Input: dimensioned drawing with shaded views. Units: mm. Origin: part minimum x, y, z. Round coordinates to 2 decimals unless told otherwise and drop trailing zeros. Loops run counter-clockwise (first coordinate to the right, second up) from the corner with the lowest first, then second, coordinate; pieces in that order, holes last. Notation, with made-up numbers: M -21.5,9.5 L 36.5,9.5 A4 ccw 36.5,14.5 Z; hole C 10,-12.5 d3. An arc over 180 degrees is marked long. Answer as CSV lines item,"result". Start each with the question number.
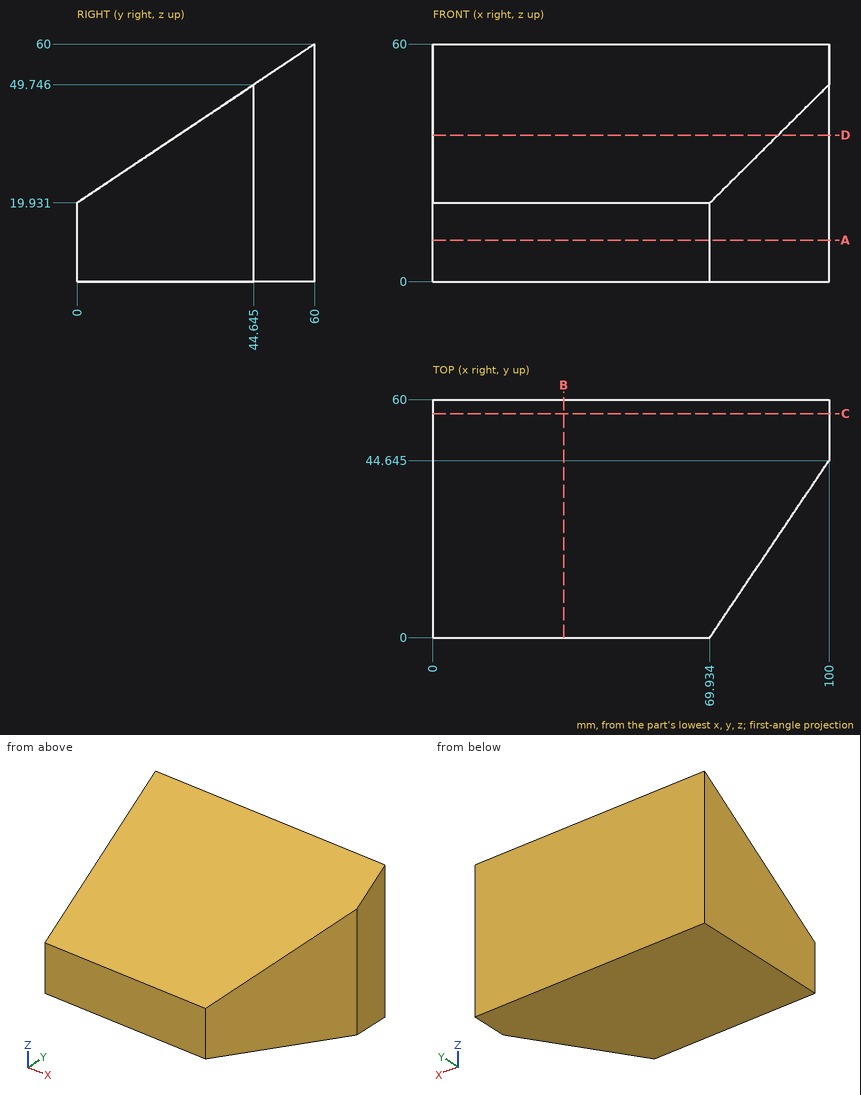
1) Section C-C, the plane y = 56.5. Return loops of the section in (x, z).
2) Contact query for flat-ended pins moving along their axis: pin 1 Ø10 at (x, z) = (16.5, 10) entering from -Y; pin 2 Ø10 at (x, y) = (54.5, 12) entering from +Z; pin 3 Ø3 at (x, y) = (11, 51.5) entering from +Z (1 decimal); pin 4 Ø2 at (x, y) = (75.5, 46) entering from +Z. Output: stop coordinate, or through.
3) Ray query, line 1 along Z through (x, y) = (60, 37); line 2 along X through (y, z) = (6, 10) (1 decimal); line 3 along Y through (x, z) = (21, 39.5) (1 decimal). Return the intervals inside material, ascending.
4) Section A-A, the plane z = 10.5. Return loops of the section in (x, y) (1 decimal).
5) Section D-D, the plane z = 37. Return loops of the section in (x, y) (1 decimal).
6) Section B-B, the plane x = 33. Return loops of the section in (y, z).
Findings below:
1,outline,"M 0,0 L 100,0 L 100,57.66 L 0,57.66 Z"
2,pin 1,"y = 0"
2,pin 2,"z = 31.28"
2,pin 3,"z = 55.3"
2,pin 4,"z = 51.32"
3,line 1,"0 to 44.64"
3,line 2,"0 to 74"
3,line 3,"29.3 to 60"
4,outline,"M 0,0 L 69.9,0 L 100,44.6 L 100,60 L 0,60 Z"
5,outline,"M 0,25.6 L 87.1,25.6 L 100,44.6 L 100,60 L 0,60 Z"
6,outline,"M 0,0 L 60,0 L 60,60 L 0,19.93 Z"
